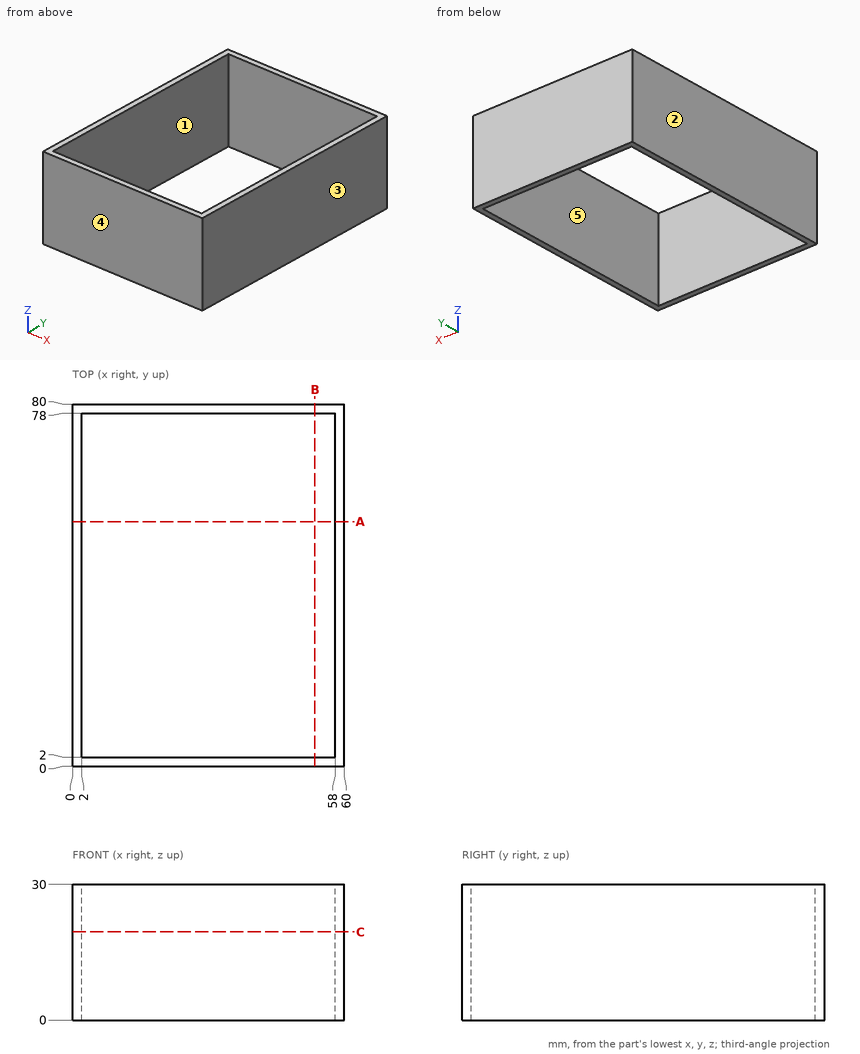
Verification items for this drawing (mm, ordinates from the low corner). A direction names the side the tool comes from. Coordinates: 2 decimals unless noted, no trailing zeros. Loops run counter-clockwise (first coordinate to the right, second up) from the corner with the lowest first, then second, coordinate; pieces in that order, holes last.
Item 1: Sectioned sample at A-A, the plane y = 54. Record the boundary of the cut face in (x, z), then the cut area to 3 significant figures.
Item 2: Thickness scan on line 1 (X direction, y = 49, z = 23.75); line 2 (Y direction, x = 16, z = 24.75). Record the ranges inside material, lowest first.
Item 3: Go/stop test with a flat-tipped pin: pin 1 Ø8 at (y, z) = (23, 14.5) entering from -X. Record where the tip stops, or that it passes through.
Item 4: Release check for a two-part mould opening along Y. For the marked faces 3, 4 and 5 record: released by +Y, released by -Y, zero draft, split by the parting line, or undercut.
Item 5: Sectioned sample at B-B, the plane x = 53.5. Record the boundary of the cut face in (y, z), then the cut area to 3 significant figures.
Item 6: Sectioned sample at C-C, the plane z = 19.5. Record the boundary of the cut face in (x, y).
Item 7: Access from +Z, -Z, +X, -X, +Y, -Y to the whole of each face (thin tool, end or side, straight path). Record for the marked faces 1 and 2.
Check result:
1. outline: (0, 0) - (2, 0) - (2, 30) - (0, 30) - close; (58, 0) - (60, 0) - (60, 30) - (58, 30) - close
1. area: 120 mm2
2. line 1: x = 0 to 2, 58 to 60
2. line 2: y = 0 to 2, 78 to 80
3. pin 1: stops at x = 0
4. face 3: zero draft
4. face 4: released by -Y
4. face 5: undercut
5. outline: (0, 0) - (2, 0) - (2, 30) - (0, 30) - close; (78, 0) - (80, 0) - (80, 30) - (78, 30) - close
5. area: 120 mm2
6. outline: (0, 0) - (60, 0) - (60, 80) - (0, 80) - close; hole (2, 2) - (58, 2) - (58, 78) - (2, 78) - close
7. face 1: +Z, -Z
7. face 2: +Z, -Z, -X, +Y, -Y
